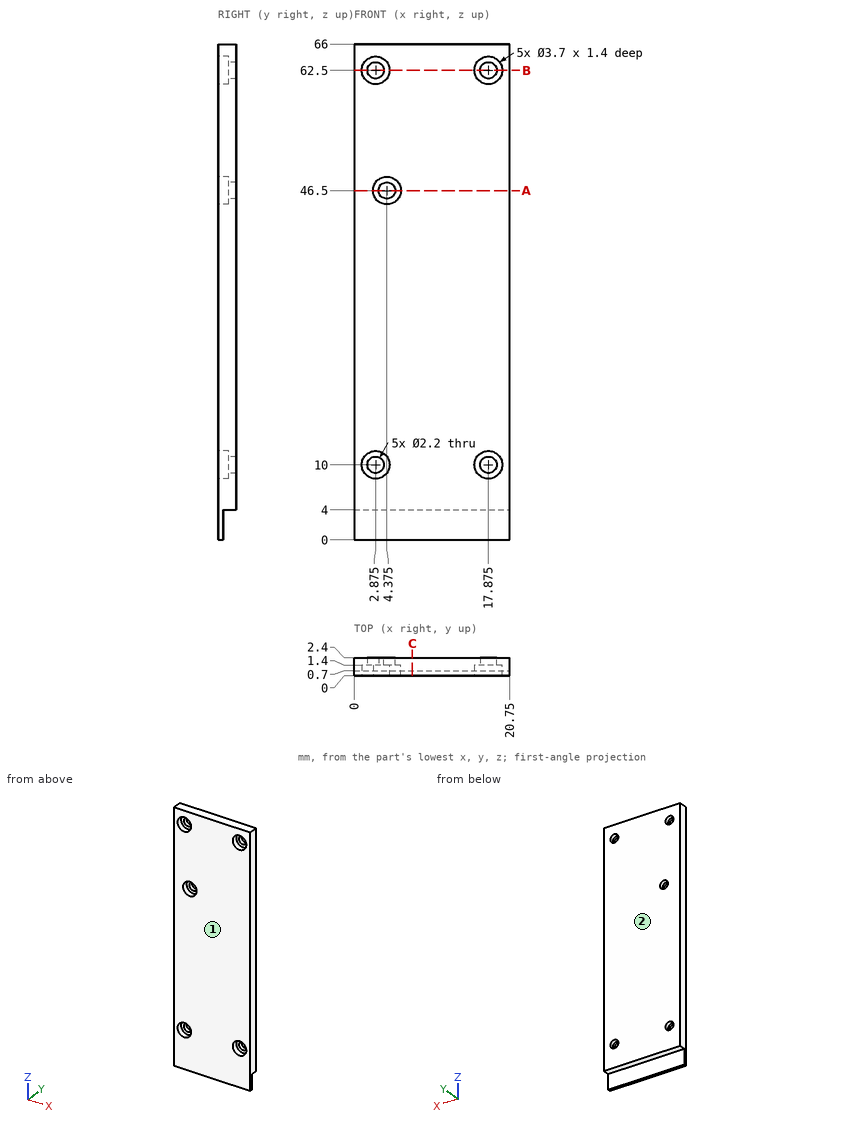
The figure shows three views and two pictorial views of one solid part (mm, origin at its lowest corner). Answer the questions. Give positions to 0.01 mm unless a question says otherwise; leave off trailing zeros. Order: outer loops, then holes, each group sorted by start corner. A loop starts at its lowest first (then second) coordinate and runs counter-clockwise, first axis right, second up. Notation, with made-up numbers: (12, -38.75) -> (50, -38.75) arc R32 cw to (50, -11.75) -> close; hole circle Ø6 at (-22, 45). An arc over 180 degrees is marked (long way). Answer as CSV lines item,"result". Start each with the question number.
Q1. Given pin 1 (1.1 mm diameter, centred on x = 17, z = 62, fed in from -Y); pin 2 (1.4 mm diameter, centred on x = 11.5, y = 1.5, fed in from -Z); pin 3 (2 mm diameter, centred on x = 12.5, z = 1.5, fed in from +Y), each flat-ended and moving along its own axis, determine where each tip first touches the part or whether it passes through.
Q2. Determine the mould class of the marked faces 1 and 2 for opening direction Y: pulls with the +Y half, pulls with the -Y half, needs draft (parallel to the pull), parting line crosses it, or undercut.
Q3. A cutting plane is placed at C-C (x = 7.75). Determine the outline of the cut face in (y, z), then the cut area to 3 significant figures.
Q4. A cutting plane is placed at B-B (z = 62.5). Determine the outline of the cut face in (x, y) (3 decimals).
Q5. Find the intervals of material crossed by L1, parallel to X at y = 2.1, z = 10 (3 decimals); L2, parallel to Z at x = 17.75, y = 2.1; L3, parallel to X at y = 0.3, z = 62.5 (3 decimals), in increasing order.
Q6. A cutting plane is placed at A-A (z = 46.5). Determine the outline of the cut face in (x, y) (3 decimals), then the cut area to 3 significant figures.
Results found:
1,pin 1,"y = 1.4"
1,pin 2,"z = 4"
1,pin 3,"y = 0.7"
2,face 1,"pulls with the -Y half"
2,face 2,"pulls with the +Y half"
3,outline,"(0, 0) -> (0.7, 0) -> (0.7, 4) -> (2.4, 4) -> (2.4, 66) -> (0, 66) -> close"
3,area,"152 mm2"
4,outline,"(0, 0) -> (1.025, 0) -> (1.025, 1.4) -> (1.775, 1.4) -> (1.775, 2.4) -> (0, 2.4) -> close; (3.975, 1.4) -> (4.725, 1.4) -> (4.725, 0) -> (16.025, 0) -> (16.025, 1.4) -> (16.775, 1.4) -> (16.775, 2.4) -> (3.975, 2.4) -> close; (18.975, 1.4) -> (19.725, 1.4) -> (19.725, 0) -> (20.75, 0) -> (20.75, 2.4) -> (18.975, 2.4) -> close"
5,L1,"0 to 1.775, 3.975 to 16.775, 18.975 to 20.75"
5,L2,"4 to 8.91, 11.09 to 61.41, 63.59 to 66"
5,L3,"0 to 1.025, 4.725 to 16.025, 19.725 to 20.75"
6,outline,"(0, 0) -> (2.525, 0) -> (2.525, 1.4) -> (3.275, 1.4) -> (3.275, 2.4) -> (0, 2.4) -> close; (5.475, 1.4) -> (6.225, 1.4) -> (6.225, 0) -> (20.75, 0) -> (20.75, 2.4) -> (5.475, 2.4) -> close"
6,area,"42.4 mm2"
